from build123d import *

# Parameters (mm, degrees)
SKETCH1_R           = 5
BOSS_EXTRUDE1_DEPTH = 3
CUT_EXTRUDE1_DEPTH  = 3
SKETCH3_R           = 4.5
CUT_EXTRUDE2_DEPTH  = 1
SKETCH27_W          = 0.25
SKETCH27_H          = 0.5


with BuildPart() as part:
    # Sketch1 → Boss-Extrude1 (new body)
    with BuildSketch(Plane(origin=(0, 0, 0), x_dir=(1, 0, 0), z_dir=(0, 1, 0))):
        with Locations(Location((0, 0, 0), (0, 0, 270))):
            Circle(SKETCH1_R)
    extrude(amount=BOSS_EXTRUDE1_DEPTH)

    # Sketch2 → Cut-Extrude1 (cut)
    with BuildSketch(Plane(origin=(0, 3, 0), x_dir=(1, 0, 0), z_dir=(0, 1, 0))):
        with BuildLine():
            ThreePointArc((3.968626967, 0.5), (2.842920112, 2.813859491), (0.540748653, 3.96328032))
            Line((0.540748653, 3.96328032), (0.540748653, 0.5))
            Line((0.540748653, 0.5), (3.968626967, 0.5))
        make_face()
        with BuildLine():
            Line((-0.5, 3.968626967), (-0.5, 0.5))
            Line((-0.5, 0.5), (-3.968626967, 0.5))
            ThreePointArc((-3.968626967, 0.5), (-2.828427125, 2.828427125), (-0.5, 3.968626967))
        make_face()
        with BuildLine():
            Line((-3.968626967, -0.5), (-0.5, -0.5))
            Line((-0.5, -0.5), (-0.5, -3.968626967))
            ThreePointArc((-0.5, -3.968626967), (-2.828427125, -2.828427125), (-3.968626967, -0.5))
        make_face()
        with BuildLine():
            Line((0.540748653, -3.96328032), (0.540748653, -0.5))
            Line((0.540748653, -0.5), (3.968626967, -0.5))
            ThreePointArc((3.968626967, -0.5), (2.842920112, -2.813859491), (0.540748653, -3.96328032))
        make_face()
    extrude(amount=-CUT_EXTRUDE1_DEPTH, mode=Mode.SUBTRACT)

    # Sketch3 → Cut-Extrude2 (cut)
    with BuildSketch(Plane(origin=(0, 3, 0), x_dir=(1, 0, 0), z_dir=(0, 1, 0))):
        with Locations(Location((0, 0, 0), (0, 0, 270))):
            Circle(SKETCH3_R)
    extrude(amount=-CUT_EXTRUDE2_DEPTH, mode=Mode.SUBTRACT)

    # Sketch22 → Revolve1 (revolve)
    with BuildSketch(Plane.XY, mode=Mode.PRIVATE) as revolve1_sk:
        Polygon((0, 4), (-0.25, 4), (-0.5, 2), (0, 2), align=None)
    revolve(revolve1_sk.sketch.rotate(Axis((0, 0, 0), (0, 1, 0)), 270), axis=Axis((0, 0, 0), (0, 1, 0)))

    # Sketch27 → Revolve2 (revolve)
    with BuildSketch(Plane.XY, mode=Mode.PRIVATE) as revolve2_sk:
        with Locations((-4.375, 2.75)):
            Rectangle(SKETCH27_W, SKETCH27_H)
    revolve(revolve2_sk.sketch.rotate(Axis((0, 2, 0), (0, 1, 0)), 90), axis=Axis((0, 2, 0), (0, 1, 0)))


solid = part.part
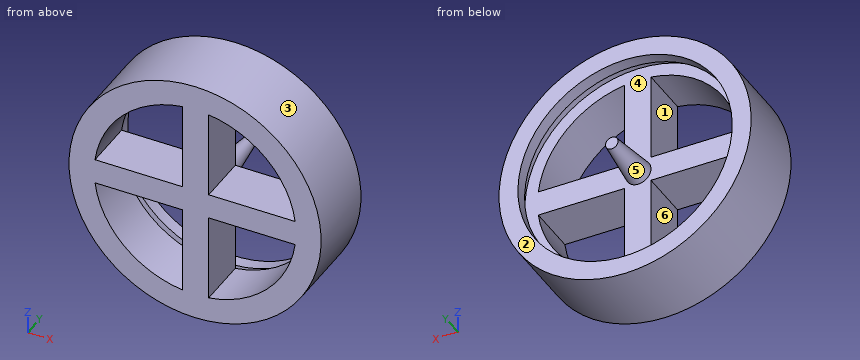
Input: part model. Units: mm. Frame: model coordinates. Face numbers are marked on the shaded views. A direction names the side the tool comes from. Round coordinates to 2 decimals unless told otherwise and drop trailing zeros. Write each loop counter-clockwise with the first axis right and the second up, starting at its lowest first coordinate (ties: lowest second). Pieces come first, ordered by that corner, then holes.
1) Cut plane C-C (x = 0). Return the cut outline in (y, z).
2) Contact query for flat-ended pins moving along their axis: P1, Ø0.6, axis at x = 3, y = 1, coming from the +Z side; P2, Ø1, axis at y = 1.5, z = 2.5, coming from the +X side; P3, Ø1, axis at x = -2.5, y = 1, coming from the +Z side. Output: stop coordinate, or through.
3) Draft query along X for the marked faces 1, 2 and 3. Return one class per face: pulls with the +X half, pulls with the -X half, needs draft (parallel to the pull), parting line crosses it, or undercut.
4) Cut plane D-D (z = 1). Return the cut outline in (x, y).
5) Reachability of the marked faces 4, 5 and 6 from +Z, -Z, +X, -X, +Y, -Y: full face, straight path, thin tool, end or side. Return the list, or none.
6) Ray query, L1, parallel to X at y = 0.4, z = -0.75; L2, parallel to X at y = 2.75, z = 0; L3, parallel to Y at x = 0.5, z = 1. Return the intervals inside material, ascending.
7) Cut plane A-A (x = 2). Return the cut outline in (y, z).
8) Cut plane B-B (z = 0). Return the cut outline in (x, y), then the cut area to 4 significant figures.
Geometry says:
1. outline: (0, -5) - (3, -5) - (3, -4.25) - (2.5, -4.25) - (2.5, -4.5) - (2, -4.5) - (2, -0.5) - (4, -0.25) - (4, 0.25) - (2, 0.5) - (2, 4.5) - (2.5, 4.5) - (2.5, 4.25) - (3, 4.25) - (3, 5) - (0, 5) - close
2. P1: stops at z = 4.21
2. P2: stops at x = 4.58
2. P3: stops at z = 4.58
3. face 1: undercut
3. face 2: needs draft
3. face 3: parting line crosses it
4. outline: (-4.9, 0) - (-3.87, 0) - (-3.87, 2) - (-4.39, 2) - (-4.39, 2.5) - (-4.13, 2.5) - (-4.13, 3) - (-4.9, 3) - close; (-0.5, 0) - (0.54, 0) - (0.54, 2) - (-0.5, 2) - close; (3.87, 0) - (4.9, 0) - (4.9, 3) - (4.13, 3) - (4.13, 2.5) - (4.39, 2.5) - (4.39, 2) - (3.87, 2) - close
5. face 4: none
5. face 5: +Y
5. face 6: +Y, -Y
6. L1: x = -4.94 to -3.93, -0.5 to 0.54, 3.93 to 4.94
6. L2: x = -5 to -4.25, -0.41 to 0.41, 4.25 to 5
6. L3: y = 0 to 2
7. outline: (0, -4.58) - (3, -4.58) - (3, -3.75) - (2.5, -3.75) - (2.5, -4.03) - (2, -4.03) - (2, -3.46) - (0, -3.46) - close; (0, -0.5) - (2, -0.5) - (2, 0.5) - (0, 0.5) - close; (0, 3.46) - (2, 3.46) - (2, 4.03) - (2.5, 4.03) - (2.5, 3.75) - (3, 3.75) - (3, 4.58) - (0, 4.58) - close
8. outline: (-5, 0) - (5, 0) - (5, 3) - (4.25, 3) - (4.25, 2.5) - (4.5, 2.5) - (4.5, 2) - (0.5, 2) - (0.25, 4) - (-0.25, 4) - (-0.5, 2) - (-4.5, 2) - (-4.5, 2.5) - (-4.25, 2.5) - (-4.25, 3) - (-5, 3) - close
8. area: 22.75 mm2
